Drawing for the job (mm, zero at the part's lowest x, y, z). A direction names the side the tool comes from. Give positions to 0.01 mm unless a question says otherwise; leave off trailing zeros. Loops run counter-clockwise (first coordinate to the right, second up) from the corner with the lowest first, then second, coordinate; pieces in that order, holes last. Notation, with made-up numbers: (-33.5, 28.25) - (-7.5, 28.25) arc R28 cw to (-7.5, 46.25) - close; hole circle Ø8 at (70.25, 88.25). An arc over 180 degrees is marked (long way). Return JSON: item names as keys, results as strings. Group by question number.
1) Slice it at C-C (y = 3.5). List the corners of the cut face in (x, z).
2) Drop flat-ended pins along their axis: pin 1 (7.5 mm diameter, centred on x = 17, y = 6.5, fed in from +Z); pin 2 (2 mm diameter, centred on y = 3.5, z = 6.84, fed in from -X). Give the stop position or say it passes through.
3) 3-axis set-ups, long thin cutter, end or side, ignore diameter. For the marked faces 1 and 2: which of +Z, -Z, +X, -X, +Y, -Y reach the whole face in a straight line?
4) Slice it at D-D (z = 6.5). List the corners of the cut face in (x, y) (1 decimal).
5) Mould opens along X. For the marked faces 3, 4 and 5 say: released by +X, released by -X, zero draft, split by the parting line, or undercut.
6) Drill centre lines: probe 1 along X at (y, z) = (7.5, 4.25); probe 2 along Z at (x, y) = (14, 5); probe 3 along Z at (x, y) = (0.5, 11.5) (1 decimal). Where is each one in solid material? Low to high. Write a range as from..to.
7) Slice it at B-B (x = 15.8). List the corners of the cut face in (y, z) (3 decimals).
8) Slice it at A-A (z = 3.75). List the corners of the cut face in (x, y).
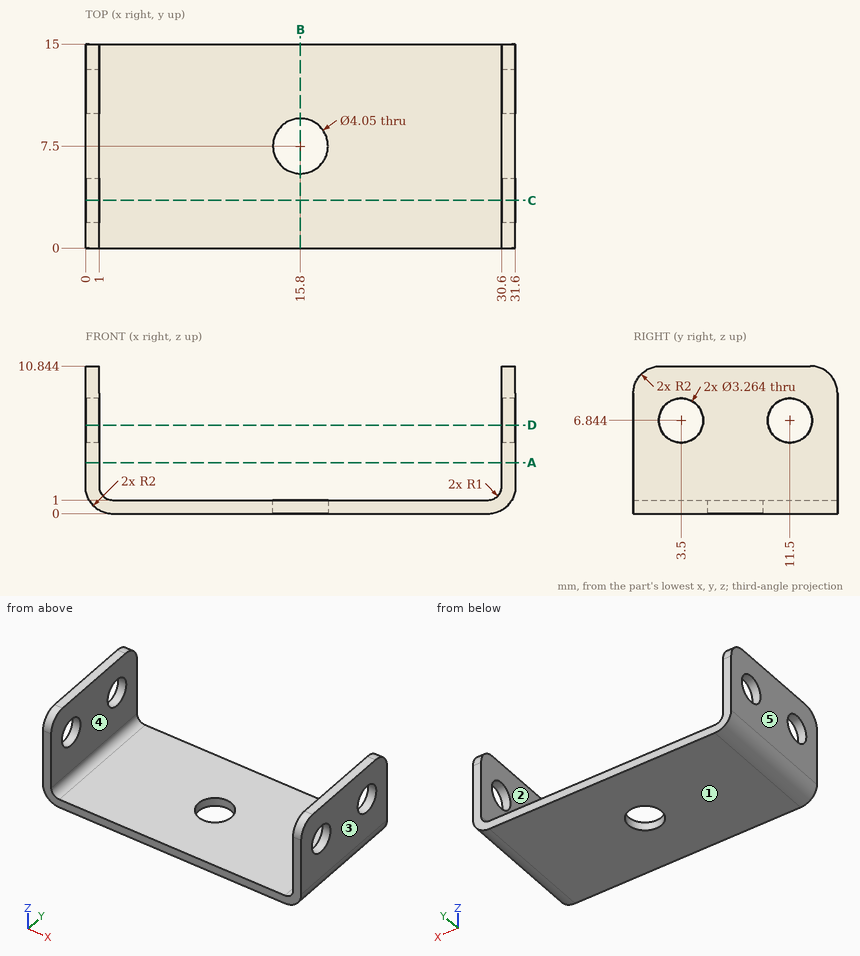
Results:
{
 "1": {"outline": "(0, 2) arc R2 ccw to (2, 0) - (29.6, 0) arc R2 ccw to (31.6, 2) - (31.6, 5.21) - (30.6, 5.21) - (30.6, 2) arc R1 cw to (29.6, 1) - (2, 1) arc R1 cw to (1, 2) - (1, 5.21) - (0, 5.21) - close; (0, 8.48) - (1, 8.48) - (1, 10.84) - (0, 10.84) - close; (30.6, 8.48) - (31.6, 8.48) - (31.6, 10.84) - (30.6, 10.84) - close"},
 "2": {"pin 1": "z = 1", "pin 2": "through"},
 "3": {"face 1": "-Z, +X, -X, +Y, -Y", "face 2": "+Z, +Y, -Y"},
 "4": {"outline": "(0, 0) - (1, 0) - (1, 1.9) - (0, 1.9) - close; (0, 5.1) - (1, 5.1) - (1, 9.9) - (0, 9.9) - close; (0, 13.1) - (1, 13.1) - (1, 15) - (0, 15) - close; (30.6, 0) - (31.6, 0) - (31.6, 1.9) - (30.6, 1.9) - close; (30.6, 5.1) - (31.6, 5.1) - (31.6, 9.9) - (30.6, 9.9) - close; (30.6, 13.1) - (31.6, 13.1) - (31.6, 15) - (30.6, 15) - close"},
 "5": {"face 3": "released by +X", "face 4": "undercut", "face 5": "released by -X"},
 "6": {"probe 1": "0..1, 30.6..31.6", "probe 2": "0..1", "probe 3": "0.7..5.2, 8.5..10.8"},
 "7": {"outline": "(0, 0) - (5.475, 0) - (5.475, 1) - (0, 1) - close; (9.525, 0) - (15, 0) - (15, 1) - (9.525, 1) - close"},
 "8": {"outline": "(0, 0) - (1, 0) - (1, 15) - (0, 15) - close; (30.6, 0) - (31.6, 0) - (31.6, 15) - (30.6, 15) - close"}
}
